```python
from build123d import *

# Parameters (mm, degrees)
SKETCH1_W           = 53.5
SKETCH1_H           = 38.5
BOSS_EXTRUDE1_DEPTH = 1.5
SKETCH2_W           = 12
SKETCH2_H           = 9.5
BOSS_EXTRUDE2_DEPTH = 4.9
FILLET1_R           = 1.5


with BuildPart() as part:
    # Sketch1 → Boss-Extrude1 (new body)
    with BuildSketch(Plane(origin=(0, 0, 0), x_dir=(1, 0, 0), z_dir=(0, 1, 0))):
        Rectangle(SKETCH1_W, SKETCH1_H)
    extrude(amount=-BOSS_EXTRUDE1_DEPTH)

    # Sketch2 → Boss-Extrude2 (add)
    # profile 1 of 2: a face of its own
    with BuildSketch(Plane(origin=(0, 0, 0), x_dir=(1, 0, 0), z_dir=(0, 1, 0))):
        with Locations((-32.75, -1.5)):
            Rectangle(SKETCH2_W, SKETCH2_H)
        Polygon((-33, -4.559956427), (-30.35, -3.029978213), (-30.35, 0.029978213), (-33, 1.559956427), (-35.65, 0.029978213), (-35.65, -3.029978213), align=None, mode=Mode.SUBTRACT)
    # profile 2 of 2: a face of its own
    with BuildSketch(Plane(origin=(0, 0, 0), x_dir=(1, 0, 0), z_dir=(0, 1, 0))):
        with Locations((32.75, -1.5)):
            Rectangle(SKETCH2_W, SKETCH2_H)
        Polygon((35.65, -3.029978213), (33, -4.559956427), (30.35, -3.029978213), (30.35, 0.029978213), (33, 1.559956427), (35.65, 0.029978213), align=None, mode=Mode.SUBTRACT)
    extrude(amount=-BOSS_EXTRUDE2_DEPTH)

    # Fillet1
    fillet1_edges = [part.edges().sort_by_distance(p)[0] for p in [
        (-26.75, -1.5, 1.5),
        (26.75, -1.5, 1.5),
    ]]
    fillet(fillet1_edges, radius=FILLET1_R)


solid = part.part
```
The model under review builds one solid part; all positions refer to its coordinate system, in mm. A direction names the side the tool comes from. Round coordinates to 2 decimals unless told otherwise and drop trailing zeros. Order: outer loops, then holes, each group sorted by start corner. A loop starts at its lowest first (then second) coordinate and runs counter-clockwise, first axis right, second up. Notation, with made-up numbers: (-38, -36.75) -> (-25, -36.75) arc R17 ccw to (-25, -17.75) -> close; hole circle Ø8 at (-16, -35.75). An arc over 180 degrees is marked (long way). Use a Markdown table: item, result.
Q1. Clearance check with flat-ended pins moving along their axes: P1, Ø1.6, axis at y = -0.5, z = -7.5, coming from the +X side; P2, Ø1.5, axis at x = 34, y = -3, coming from the +Z side; P3, Ø12, axis at x = -23.5, z = 1.5, coming from the +Y side; P4, Ø0.8, axis at y = -1, z = -12.5, coming from the -X side. State where each tip first meets the part, or that it passes through.
Values:
| item | result |
|---|---|
| P1 | stops at x = 26.75 |
| P2 | stops at z = 6.25 |
| P3 | stops at y = 0 |
| P4 | stops at x = -26.75 |
Q2. Tool access review of faces 5 (the cylindrical face through (26.3, -1.93, 1.43)), 6 (the flat face through (26.75, -1, 13)), 7 (the flat face through (34.306, -2.416, -0.806)): name each direction out of +Z, -Z, +X, -X, +Y, -Y from which nothing blocks a thin tool from reaching the whole face with its end or side.
Values:
| item | result |
|---|---|
| face 5 | +Z, -Z, -Y |
| face 6 | +Z, +X, +Y, -Y |
| face 7 | +Y, -Y |
Q3. For line 1 (X direction, y = -0.6, z = 1.5); line 2 (Y direction, x = -7, z = -5.5); line 3 (X direction, y = -3, z = 5), list the stretches that pass through material, from the lowest coordinate up.
Values:
| item | result |
|---|---|
| line 1 | x = -38.75 to -35.65, -30.35 to 30.35, 35.65 to 38.75 |
| line 2 | y = -1.5 to 0 |
| line 3 | x = -38.75 to -26.75, 26.75 to 38.75 |
Q4. We need section C-C on x = -6.5. Write out the cut boundary in (y, z), then the cut area to 4 significant figures.
Values:
| item | result |
|---|---|
| outline | (-1.5, -19.25) -> (0, -19.25) -> (0, 19.25) -> (-1.5, 19.25) -> close |
| area | 57.75 mm^2 |
Q5. We need section B-B on z = 16.5. Write out the cut boundary in (x, y), then the cut area to 4 significant figures.
Values:
| item | result |
|---|---|
| outline | (-26.75, -1.5) -> (26.75, -1.5) -> (26.75, 0) -> (-26.75, 0) -> close |
| area | 80.25 mm^2 |
Q6. We need section A-A on y = -2.2. Write out the cut boundary in (x, z), then the cut area to 3 significant figures.
Values:
| item | result |
|---|---|
| outline | (-38.75, -3.25) -> (-26.52, -3.25) -> (-26.52, 6.25) -> (-38.75, 6.25) -> close; (26.52, -3.25) -> (38.75, -3.25) -> (38.75, 6.25) -> (26.52, 6.25) -> close; hole (-35.65, -0.03) -> (-33, -1.56) -> (-30.35, -0.03) -> (-30.35, 3.03) -> (-33, 4.56) -> (-35.65, 3.03) -> close; hole (30.35, -0.03) -> (33, -1.56) -> (35.65, -0.03) -> (35.65, 3.03) -> (33, 4.56) -> (30.35, 3.03) -> close |
| area | 184 mm^2 |
Q7. Mouldability with a two-part tool opening along X and no side actions: class faces 1 (the flat face through (38.75, -2, 2)), 2 (the flat face through (33, -2, 6.25)), 3 (the flat face through (31.694, -2.416, 3.806)), 4 (the flat face through (-38.75, -2, 2)) as +X half, -X half, draft (parallel to the pull), parting line (faces both ways), or undercut.
Values:
| item | result |
|---|---|
| face 1 | +X half |
| face 2 | draft |
| face 3 | undercut |
| face 4 | -X half |
